Check sheet for the modelled part. Datum: model origin and axes. Units: mm. A direction names the side the tool comes from. Round coordinates to 2 decimals unless told otherwise and drop trailing zeros. Order: outer loops, then holes, each group sorted by start corner. A loop starts at its lowest first (then second) coordinate and runs counter-clockwise, first axis right, second up.
```python
from build123d import *

# Parameters (mm, degrees)
SKETCH_2_W           = 30.5
SKETCH_2_H           = 20.5
SKETCH_2_W_2         = 22.5
SKETCH_2_H_2         = 12.5
EXTRUDE_1_DEPTH      = 12
SKETCH_3_W           = 2.75
SKETCH_3_H           = 10
EXTRUDE_2_DEPTH      = 3
SKETCH_4_W           = 4.940698383
SKETCH_4_H           = 10
CUT_EXTRUDE_1_DEPTH  = 9
EXTRUDE_3_DEPTH      = 20
EXTRUDE_4_REACH      = 38.805
SKETCH_7_R           = 0.75
CUT_EXTRUDE_2_DEPTH  = 41.374032496
SKETCH_8_W           = 10
SKETCH_8_H           = 10
CUT_EXTRUDE_3_DEPTH  = 18
SKETCH_10_W          = 23.106147985
SKETCH_10_H          = 7.754593222
CUT_EXTRUDE_4_DEPTH  = 42.146840705
SKETCH_11_R          = 1.5
CUT_EXTRUDE_5_DEPTH  = 44.934610502
CUT_EXTRUDE_6_REACH  = 60.181
SKETCH_12_W          = 11
SKETCH_12_H          = 11
SKETCH_13_W          = 23.5
SKETCH_13_H          = 13.5
CUT_EXTRUDE_7_DEPTH  = 42.146840705
SKETCH_14_W          = 9.129424231
SKETCH_14_H          = 10.218893611
CUT_EXTRUDE_8_DEPTH  = 42.146840705
CUT_EXTRUDE_9_REACH  = 45.935
CUT_EXTRUDE_10_REACH = 43.147
SKETCH_16_R          = 1.5
SKETCH_17_W          = 5.816970736
SKETCH_17_H          = 10.394960723
EXTRUDE_5_DEPTH      = 3


with BuildPart() as part:
    # 草图2 → 凸台-拉伸1 (new body)
    with BuildSketch(Plane.XY):
        Rectangle(SKETCH_2_W, SKETCH_2_H)
        Rectangle(SKETCH_2_W_2, SKETCH_2_H_2, mode=Mode.SUBTRACT)
    extrude(amount=EXTRUDE_1_DEPTH)

    # 草图3 → 凸台-拉伸2 (add)
    with BuildSketch(Plane.XY.offset(12)):
        with Locations((-16.625, 0)):
            Rectangle(SKETCH_3_W, SKETCH_3_H)
    extrude_2 = extrude(amount=-EXTRUDE_2_DEPTH)

    # 镜向1: 凸台-拉伸2 across plane
    add(extrude_2.mirror(Plane(origin=(0, 0, 0), x_dir=(0, 0, 1), z_dir=(1, 0, 0))))

    # 草图4 → 切除-拉伸1 (cut)
    with BuildSketch(Plane(origin=(0, 0, 0), x_dir=(-1, 0, 0), z_dir=(0, 0, -1))):
        with Locations((15.220349192, 0)):
            Rectangle(SKETCH_4_W, SKETCH_4_H)
    cut_extrude_1 = extrude(amount=-CUT_EXTRUDE_1_DEPTH, mode=Mode.SUBTRACT)

    # 镜向2: 切除-拉伸1 across plane
    add(cut_extrude_1.mirror(Plane(origin=(0, 0, 0), x_dir=(0, 0, 1), z_dir=(1, 0, 0))), mode=Mode.SUBTRACT)

    # 草图5 → 凸台-拉伸3 (add)
    with BuildSketch(Plane.ZY.offset(18)):
        Polygon((12, 10.25), (12, 5), (12, -5), (12, -10.25), (0, -10.25), (0, -5), (0, 5), (0, 10.25), align=None)
    extrude(amount=EXTRUDE_3_DEPTH)

    # 草图6 → 凸台-拉伸4 (add, up to next)
    with BuildSketch(Plane.ZY.offset(15.25), mode=Mode.PRIVATE) as extrude_4_sk1:
        Polygon((12, -5), (9, -5), (0, -5), (0, -10.25), (12, -10.25), align=None)
    extrude_4_tool1 = extrude(extrude_4_sk1.sketch, amount=EXTRUDE_4_REACH, mode=Mode.PRIVATE) - part.part
    extrude_4 = extrude_4_tool1.solids().sort_by_distance((-15.25, -7.625, 6))[0]
    add(extrude_4)

    # 镜向3: 凸台-拉伸4 across plane
    add(extrude_4.mirror(Plane.ZX))

    # 草图7 → 切除-拉伸2 (cut, through all)
    with BuildSketch(Plane(origin=(0, 0, 9), x_dir=(-1, 0, 0), z_dir=(0, 0, -1))):
        with Locations((14.25, 0)):
            Circle(SKETCH_7_R)
    cut_extrude_2 = extrude(amount=-CUT_EXTRUDE_2_DEPTH, mode=Mode.SUBTRACT)

    # 草图8 → 切除-拉伸3 (cut)
    with BuildSketch(Plane.ZY.offset(38)):
        with Locations((6, 0)):
            Rectangle(SKETCH_8_W, SKETCH_8_H)
    extrude(amount=-CUT_EXTRUDE_3_DEPTH, mode=Mode.SUBTRACT)

    # 草图10 → 切除-拉伸4 (cut, through all)
    with BuildSketch(Plane(origin=(0, 0, 0), x_dir=(-1, 0, 0), z_dir=(0, 0, -1))):
        with Locations((31.553073992, 12.127296611)):
            Rectangle(SKETCH_10_W, SKETCH_10_H)
    cut_extrude_4 = extrude(amount=-CUT_EXTRUDE_4_DEPTH, mode=Mode.SUBTRACT)

    # 镜向4: 切除-拉伸4 across plane
    add(cut_extrude_4.mirror(Plane.ZX), mode=Mode.SUBTRACT)

    # 草图11 → 切除-拉伸5 (cut, through all)
    with BuildSketch(Plane.XZ.offset(8.25)):
        with Locations(Location((-28, 6, 0), (0, 0, 270))):
            Circle(SKETCH_11_R)
    extrude(amount=-CUT_EXTRUDE_5_DEPTH, mode=Mode.SUBTRACT)

    # 镜向5: 切除-拉伸2 across plane
    add(cut_extrude_2.mirror(Plane(origin=(0, 0, 0), x_dir=(0, 0, 1), z_dir=(1, 0, 0))), mode=Mode.SUBTRACT)

    # 切除-拉伸6: up to this face of the body (flat: up to its plane)
    cut_extrude_6_end = Plane(part.part.faces().sort_by_distance((-20, 0, 6))[0])
    # 草图12 → 切除-拉伸6 (cut, up to the picked face)
    with BuildSketch(Plane.ZY.offset(38), mode=Mode.PRIVATE) as cut_extrude_6_sk1:
        with Locations((6, 0)):
            Rectangle(SKETCH_12_W, SKETCH_12_H)
    cut_extrude_6_tool1 = split(extrude(cut_extrude_6_sk1.sketch, amount=-CUT_EXTRUDE_6_REACH, mode=Mode.PRIVATE), bisect_by=cut_extrude_6_end, keep=Keep.BOTH, mode=Mode.PRIVATE)
    add(cut_extrude_6_tool1.solids().sort_by(Axis((-38, 0, 6), (1, 0, 0)))[0], mode=Mode.SUBTRACT)

    # 草图13 → 切除-拉伸7 (cut, through all)
    with BuildSketch(Plane.XY.offset(12)):
        Rectangle(SKETCH_13_W, SKETCH_13_H)
    extrude(amount=-CUT_EXTRUDE_7_DEPTH, mode=Mode.SUBTRACT)

    # 草图14 → 切除-拉伸8 (cut, through all)
    with BuildSketch(Plane.XY.offset(12)):
        with Locations((13.435287884, 0.109446806)):
            Rectangle(SKETCH_14_W, SKETCH_14_H)
    extrude(amount=-CUT_EXTRUDE_8_DEPTH, mode=Mode.SUBTRACT)

    # 草图15 → 切除-拉伸9 (cut, up to next)
    with BuildSketch(Plane(origin=(0, 8.25, 0), x_dir=(1, 0, 0), z_dir=(0, 1, 0)), mode=Mode.PRIVATE) as cut_extrude_9_sk1:
        Polygon((-24.535898385, -6), (-26.267949192, -3), (-29.732050808, -3), (-31.464101615, -6), (-29.732050808, -9), (-26.267949192, -9), align=None)
    cut_extrude_9_tool1 = extrude(cut_extrude_9_sk1.sketch, amount=-CUT_EXTRUDE_9_REACH, mode=Mode.PRIVATE) & part.part
    add(cut_extrude_9_tool1.solids().sort_by_distance((-28, 8.25, 6))[0], mode=Mode.SUBTRACT)

    # 草图16 → 切除-拉伸10 (cut, up to next)
    with BuildSketch(Plane(origin=(0, 0, 0), x_dir=(-1, 0, 0), z_dir=(0, 0, -1)), mode=Mode.PRIVATE) as cut_extrude_10_sk1:
        with Locations((28, 0)):
            Circle(SKETCH_16_R)
    cut_extrude_10_tool1 = extrude(cut_extrude_10_sk1.sketch, amount=-CUT_EXTRUDE_10_REACH, mode=Mode.PRIVATE) & part.part
    add(cut_extrude_10_tool1.solids().sort_by_distance((-28, 0, 0))[0], mode=Mode.SUBTRACT)

    # 草图17 → 凸台-拉伸5 (add)
    with BuildSketch(Plane.XY.offset(12)):
        with Locations((14.658485368, 0.02141325)):
            Rectangle(SKETCH_17_W, SKETCH_17_H)
    extrude(amount=-EXTRUDE_5_DEPTH)

    # 镜向6: 切除-拉伸2 across plane
    add(cut_extrude_2.mirror(Plane.ZY), mode=Mode.SUBTRACT)


solid = part.part
```
Item 1: Sectioned sample at A-A (x = 14.25). Record the cut outline in (y, z), and give its area (3 significant figures).
Answer:
outline: (-10.25, 0) - (-5, 0) - (-5, 9) - (-0.75, 9) - (-0.75, 12) - (-10.25, 12) - close; (0.75, 9) - (5.22, 9) - (5.22, 0) - (10.25, 0) - (10.25, 12) - (0.75, 12) - close
area: 150 mm2
Item 2: Release check for a two-part mould opening along X. For faces 1 (the flat face through (-28, 7, 9)), 2 (the flat face through (-29.1, -1.3, 0.5)), 3 (the flat face through (-38, 6, 7)) record: released by +X, released by -X, zero draft, split by the parting line, or undercut.
Answer:
face 1: undercut
face 2: zero draft
face 3: released by -X
Item 3: Sectioned sample at D-D (z = 1.5). Record the cut outline in (x, y).
Answer:
outline: (-38, -8.25) - (-20, -8.25) - (-20, -10.25) - (15.25, -10.25) - (15.25, -5) - (11.75, -5) - (11.75, -6.75) - (-11.75, -6.75) - (-11.75, 6.75) - (11.75, 6.75) - (11.75, 5.22) - (15.25, 5.22) - (15.25, 10.25) - (-20, 10.25) - (-20, 8.25) - (-38, 8.25) - (-38, 5.5) - (-20, 5.5) - (-20, -5.5) - (-38, -5.5) - close; hole (-18, -5) - (-12.75, -5) - (-12.75, 5) - (-18, 5) - close
Item 4: Sectioned sample at C-C (y = 4.5). Record the cut outline in (x, z), and give its area (3 significant figures).
Answer:
outline: (-38, 0) - (-18, 0) - (-18, 9) - (-12.75, 9) - (-12.75, 0) - (-11.75, 0) - (-11.75, 12) - (-38, 12) - (-38, 11.5) - (-20, 11.5) - (-20, 0.5) - (-38, 0.5) - close; (11.75, 9) - (17.57, 9) - (17.57, 12) - (11.75, 12) - close
area: 87.2 mm2
Item 5: Access from +Z, -Z, +X, -X, +Y, -Y to the whole of each face (thin tool, end or side, straight path). Record for faces 4 (the flat face through (15.25, 8, 6)), 5 (the flat face through (-12.75, 0, 4)), 6 (the flat face through (-31.1, 5.5, 7.1)), 7 (the flat face through (-28.9, -8.25, 4.6)).
Answer:
face 4: +Z, -Z, +X, +Y
face 5: -Z
face 6: -X
face 7: +Z, -Z, -X, -Y
Item 6: Scan lines: line 1 along X through (y, z) = (-5.75, 10.5); line 2 along Y through (x, z) = (-14.25, 10.25); line 3 along Z through (x, y) = (-25, -1.25). Record each from-to range of solid material in increasing order.
Answer:
line 1: x = -38 to -11.75, 11.75 to 15.25
line 2: y = -10.25 to -0.75, 0.75 to 10.25
line 3: z = 0 to 0.5, 11.5 to 12
Item 7: Sectioned sample at B-B (z = 5). State how many separate pieces and enclosed holes the cut face has, and give its area (3 significant figures).
Answer:
separate pieces: 3
enclosed holes: 1
area: 394 mm2
Item 8: Go/stop test with flat-tipped pins: P1, Ø6, axis at y = -0.5, z = 3, coming from the +X side; P2, Ø1.5, axis at y = -5.5, z = 1.5, coming from the +X side; P3, Ø1.8, axis at x = -28, y = 0, coming from the -Z side. Record where each tip stops, or that it passes through.
Answer:
P1: stops at x = -11.75
P2: stops at x = 15.25
P3: stops at z = 11.5
